Can you work these out from the model? Positions are in its coordinate system, mm. A direction names the side the tool comes from. Give positions to 0.01 mm unless a question says otherwise; leave off trailing zeros. Order: outer loops, then holes, each group sorted by start corner. A loop starts at its lowest first (then second) coordinate and runs counter-clockwise, first axis right, second up. Notation, with made-up numbers: M 18,-24 L 71,-24 A24 ccw 71,0 Z; hole C 26.25,32 d5. An arc over 180 degrees is marked long. Use one line per item in the form item = value. Start each with the question number.
1. I want a section at A-A, the plane x = 38. List the corners of the cut face in (y, z) for me, and give its area (3 significant figures).
2. I want a section at C-C, the plane x = 67. List the corners of the cut face in (y, z) for me.
3. I need wall thicknesses on L1, parallel to Z at x = 22, y = -3.6; L2, parallel to Z at x = 32, y = 2.25; L3, parallel to Y at x = 83.5, z = 3. Which ranges of each line are inside material? Lowest first, please.
4. We'd pull the mould along X, two halves only. Please class faces 1 (the face through (55.43, -3.03, 0.45)), 2 (the face through (-3, 2, 0)), 3 (the face through (49, 5, 7)): +X half, -X half, draft (parallel to the pull), parting line (faces both ways), or undercut.
5. I want a section at B-B, the plane y = -2.75. Count the separate pieces of the cut face and the enclosed holes in it, and give its area (3 significant figures).
6. Will these pins go through, and if not, where does the flat tip stop? P1, Ø4, axis at x = 43.5, y = 7.5, coming from the +Z side; P2, Ø6, axis at y = 0, z = 0.5, coming from the +X side; P3, Ø3, axis at x = 33, z = 8, coming from the +Y side; P4, Ø2, axis at y = 6.5, z = -6, coming from the +X side.
7. For faces 4 (the face through (49.3, 1.958, 5.107)), 5 (the face through (49, 5, -7)), 6 (the face through (48, 0, 10)), which set-ups out of +Z, -Z, +X, -X, +Y, -Y let a thin tool reach every point of the face, with its end or its side?
Autodesk Inventor part; units mm, degrees
ref_plane "YZ Plane" through (0, 0, 0) normal (1, 0, 0) x (0, 1, 0)
ref_plane "XZ Plane" through (0, 0, 0) normal (0, 1, 0) x (-1, 0, 0)
ref_plane "XY Plane" through (0, 0, 0) normal (0, 0, 1) x (1, 0, 0)
sketch "Sketch1" plane through (0, 0, 0) normal (1, 0, 0) x (0, 1, 0)
  line L0 (-5, 10) -> (5, 10)
  line L1 (5, 10) -> (5, -10)
  line L2 (5, -10) -> (-5, -10)
  line L3 (-5, -10) -> (-5, 10)
  line L4 (-5, 10) -> (5, -10) construction
  line L5 (5, 10) -> (-5, -10) construction
  line L6 (-1, 6.1838) -> (-1, -6.1838)
  line L7 (-1, -6.1838) -> (5, -4)
  line L8 (-1, 6.1838) -> (5, 4)
  point P0 (0, 0)
  dimension "d0" = 10
  dimension "d1" = 20
  dimension "d3" = 110
  dimension "d4" = 110
  dimension "d5" = 6
  dimension "d6" = 6
  dimension "d7" = 6
  dimension "d8" = 6
extrude "Extrusion1" add sketch "Sketch1" along normal blind 100 contours L0 L1 L8 L6 L7 L2 L3
sketch "Sketch2" plane through (0, 0, 0) normal (-1, 0, 0) x (0, 0, 1)
  line L0 (-10, -5) -> (-10, 5)
  line L1 (-10, -5) -> (10, -5)
  line L2 (10, -5) -> (10, 9)
  line L3 (10, 9) -> (-10, 9)
  line L4 (-10, 9) -> (-10, -5)
  point P0 (0, 0)
  dimension "d11" = 20
  dimension "d12" = 14
extrude "Extrusion2" add sketch "Sketch2" along normal blind 3
sketch "Sketch3" plane through (100, -5, -10) normal (0, -1, 0) x (1, 0, 0)
  circle A0 centre (-6, 10) radius 1.5
  circle A1 centre (-14, 10) radius 1.5
  circle A2 centre (-22, 10) radius 1.5
  circle A3 centre (-30, 10) radius 1.5
  circle A4 centre (-38, 10) radius 1.5
  circle A5 centre (-46, 10) radius 1.5
  circle A6 centre (-54, 10) radius 1.5
  line L0 (-103, 0) -> (0, 0)
  line L1 (0, 20) -> (0, 0)
  line L2 (0, 20) -> (-103, 20)
  line L3 (-103, 0) -> (-103, 20)
  circle A7 centre (-62, 10) radius 1.5
  circle A8 centre (-70, 10) radius 1.5
  circle A9 centre (-78, 10) radius 1.5
  circle A10 centre (-86, 10) radius 1.5
  circle A11 centre (-94, 10) radius 1.5
  point P0 (-100, 10)
extrude "Extrusion3" cut sketch "Sketch3" against normal through all contours A0 | A1 | A2 | A3 | A4 | A5 | A6 | A7 | A8 | A9 | A10 | A11
properties part number "prismatic link inner"
Check result:
q1.outline = M -5,-10 L 5,-10 L 5,-4 L -1,-6.18 L -1,-1.5 L -5,-1.5 Z; M -5,1.5 L -1,1.5 L -1,6.18 L 5,4 L 5,10 L -5,10 Z
q1.area = 127 mm2
q2.outline = M -5,-10 L 5,-10 L 5,-4 L -1,-6.18 L -1,6.18 L 5,4 L 5,10 L -5,10 Z
q3.L1 = -10 to -1.5, 1.5 to 10
q3.L2 = -10 to -5, 5 to 10
q3.L3 = -5 to -1
q4.face_1 = undercut
q4.face_2 = -X half
q4.face_3 = draft
q5.separate_pieces = 1
q5.enclosed_holes = 12
q5.area = 1,980 mm2
q6.P1 = through
q6.P2 = 100
q6.P3 = 5
q6.P4 = 0
q7.face_4 = +X
q7.face_5 = +Z, -Z, +X, +Y
q7.face_6 = +Z, +X, -X, +Y, -Y
